For this review, use the dimensioned drawing (mm, ordinates from the lowest corner) and the shaded views. A direction names the side the tool comes from. Give positions to 0.01 mm unless a question says otherwise; leave off trailing zeros. Order: outer loops, then holes, each group sorted by start corner. A loop starts at its lowest first (then second) coordinate and runs counter-clockwise, first axis right, second up. Notation, with made-up numbers: M -6,37.25 L 5,37.25 A14 ccw 5,63.25 Z; hole C 73.25,-27.75 d9. An arc over 180 degrees is marked long. Answer as CSV lines item,"result". Start each with the question number.
1. For line 1 along Y through (x, z) = (9.5, 43.95); line 2 along X through (y, z) = (1, 22); line 3 along Y through (x, z) = (25, 44), list the stretches that pass through material, from the lowest coordinate up.
2. Clearance check with flat-ended pins moving along their axes: P1, Ø15, axis at x = 30.5, y = 26, coming from the -Z side; P2, Ø8, axis at x = 28.5, z = 22, coming from the +Y side. State where each tip first meets the part, or that it passes through.
3. We need section C-C, the plane z = 22. Give the boundary of the cut face in (x, y).
4. We need section D-D, the plane x = 9.5. Give the boundary of the cut face in (y, z).
5. Machinability: for the marked faces 1 and 2, which of the approach directions +Z, -Z, +X, -X, +Y, -Y give a long, thin tool a straight path to every point of the face, cutting with its end or side? Answer none if there is none.
6. We need section A-A, the plane y = 19.5. Give the boundary of the cut face in (x, z).
7. We need section B-B, the plane x = 25. Give the boundary of the cut face in (y, z), and give its area (3 significant figures).
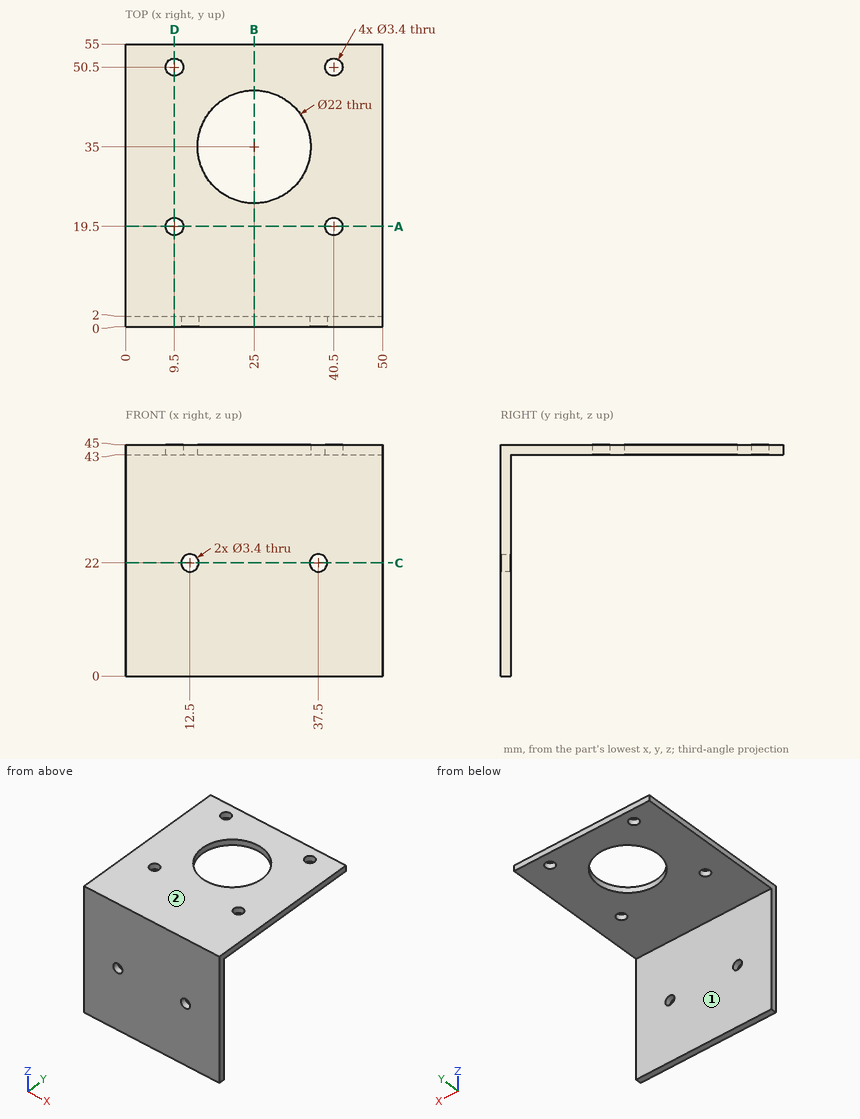
Result set:
1,line 1,"0 to 17.8, 21.2 to 48.8, 52.2 to 55"
1,line 2,"0 to 10.8, 14.2 to 35.8, 39.2 to 50"
1,line 3,"0 to 24, 46 to 55"
2,P1,"z = 43"
2,P2,"y = 2"
3,outline,"M 0,0 L 10.8,0 L 10.8,2 L 0,2 Z; M 14.2,0 L 35.8,0 L 35.8,2 L 14.2,2 Z; M 39.2,0 L 50,0 L 50,2 L 39.2,2 Z"
4,outline,"M 0,0 L 2,0 L 2,43 L 17.8,43 L 17.8,45 L 0,45 Z; M 21.2,43 L 48.8,43 L 48.8,45 L 21.2,45 Z; M 52.2,43 L 55,43 L 55,45 L 52.2,45 Z"
5,face 1,"-Z, +X, -X, +Y"
5,face 2,"+Z, +X, -X, +Y, -Y"
6,outline,"M 0,43 L 7.8,43 L 7.8,45 L 0,45 Z; M 11.2,43 L 38.8,43 L 38.8,45 L 11.2,45 Z; M 42.2,43 L 50,43 L 50,45 L 42.2,45 Z"
7,outline,"M 0,0 L 2,0 L 2,43 L 24,43 L 24,45 L 0,45 Z; M 46,43 L 55,43 L 55,45 L 46,45 Z"
7,area,"152 mm2"
